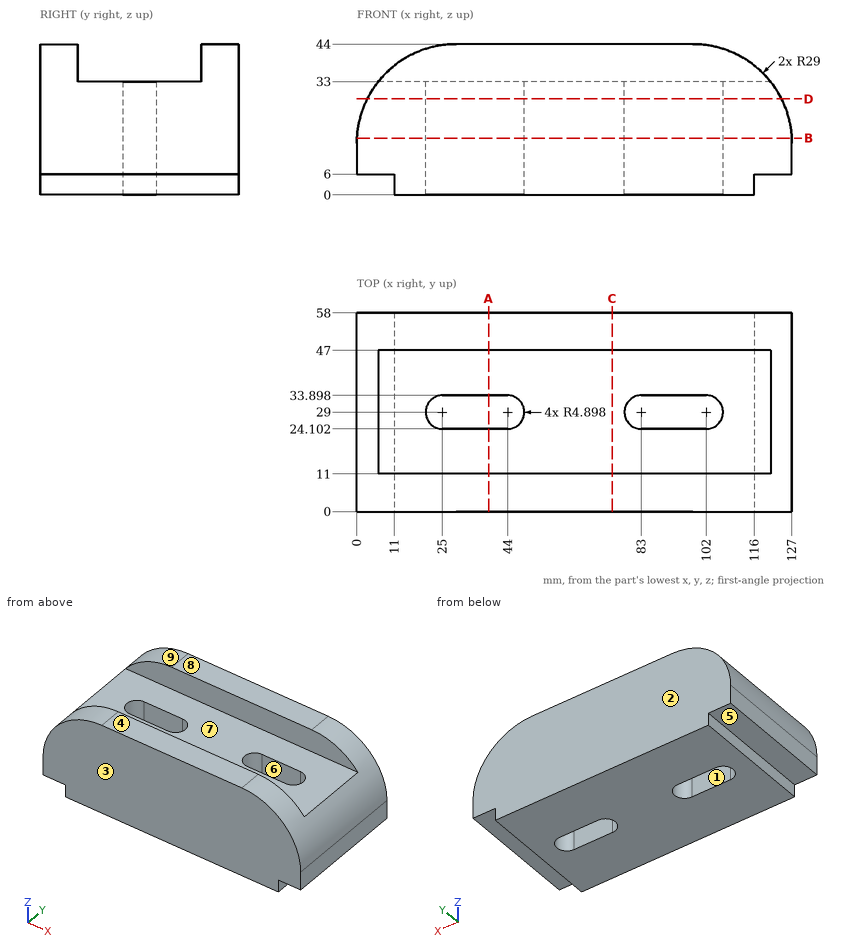
Geometry check sheet. Reference: drawing and pictorial views, mm from the part's lowest x, y, z. A direction names the side the tool comes from. Give positions to 0.01 mm unless a question says otherwise; leave off trailing zeros. Order: outer loops, then holes, each group sorted by start corner. A loop starts at its lowest first (then second) coordinate and runs counter-clockwise, first axis right, second up. Notation, with made-up numbers: (69.25, 47.25) - (81.25, 47.25) arc R25 cw to (81.25, 85.25) - close; hole circle Ø5 at (-30.75, 82). An arc over 180 degrees is marked (long way). Use one line per item in the form item = value.
1) Sectioned sample at B-B (z = 16.5). Record the boundary of the cut face in (x, y), and give its area (3 significant figures).
Working result:
outline = (0.04, 0) - (126.96, 0) - (126.96, 58) - (0.04, 58) - close; hole (25, 24.1) - (44, 24.1) arc R4.9 ccw to (44, 33.9) - (25, 33.9) arc R4.9 ccw to start; hole (83, 24.1) - (102, 24.1) arc R4.9 ccw to (102, 33.9) - (83, 33.9) arc R4.9 ccw to start
area = 6,840 mm^2
2) Sectioned sample at A-A (x = 38.5). Record the boundary of the cut face in (y, z), and give its area (3 significant figures).
Working result:
outline = (0, 0) - (24.1, 0) - (24.1, 33) - (11, 33) - (11, 44) - (0, 44) - close; (33.9, 0) - (58, 0) - (58, 44) - (47, 44) - (47, 33) - (33.9, 33) - close
area = 1,830 mm^2
3) Material ranges on probe 1 along X at (y, z) = (25.5, 22.5) (1 decimal); probe 2 along Y at (x, z) = (68.5, 38); probe 3 along Y at (x, z) = (96.5, 10), recorded low to high. Write a range as from..to.
Working result:
probe_1 = 1..21.6, 47.4..79.6, 105.4..126
probe_2 = 0..11, 47..58
probe_3 = 0..24.1, 33.9..58
4) Depth check by flat-ended pin: pin 1 Ø6.5 at (y, z) = (30.5, 2) entering from +X; pin 2 Ø8 at (x, y) = (35.5, 42) entering from +Z; pin 3 Ø6.5 at (y, z) = (29.5, 2.5) entering from -X. Enter the tip coordinate at first touch or a pass-through.
Working result:
pin_1 = 116
pin_2 = 33
pin_3 = 11
5) Sectioned sample at D-D (z = 28). Record the boundary of the cut face in (x, y), and give its area (3 significant figures).
Working result:
outline = (3.08, 0) - (123.92, 0) - (123.92, 58) - (3.08, 58) - close; hole (25, 24.1) - (44, 24.1) arc R4.9 ccw to (44, 33.9) - (25, 33.9) arc R4.9 ccw to start; hole (83, 24.1) - (102, 24.1) arc R4.9 ccw to (102, 33.9) - (83, 33.9) arc R4.9 ccw to start
area = 6,490 mm^2
6) Draft check along Y on the marked faces 1, 2, 3 and 4. Enter one of: released by +Y, released by -Y, zero draft, split by the parting line, or undercut.
Working result:
face_1 = undercut
face_2 = released by +Y
face_3 = released by -Y
face_4 = zero draft
7) Sectioned sample at C-C (x = 74.5). Record the boundary of the cut face in (y, z), and give its area (3 significant figures).
Working result:
outline = (0, 0) - (58, 0) - (58, 44) - (47, 44) - (47, 33) - (11, 33) - (11, 44) - (0, 44) - close
area = 2,160 mm^2
8) Access from +Z, -Z, +X, -X, +Y, -Y to the whole of each face (thin tool, end or side, straight path). Record for the marked faces 5, 6, 7, 8 and 9.
Working result:
face_5 = -Z, -X, +Y, -Y
face_6 = +Z, -Z
face_7 = +Z, +X, -X
face_8 = +Z, +X, -X, +Y, -Y
face_9 = +Z, -X, +Y, -Y
